Verification items for the finished model (mm, model axes). Face numbers are marked on the shaded views. Give positions to 0.01 mm unless a question says otherwise; leave off trailing zeros. Write each loop counter-clockwise with the first axis right and the second up, starting at its lowest first coordinate (ties: lowest second). Pieces come first, ordered by that corner, then holes.
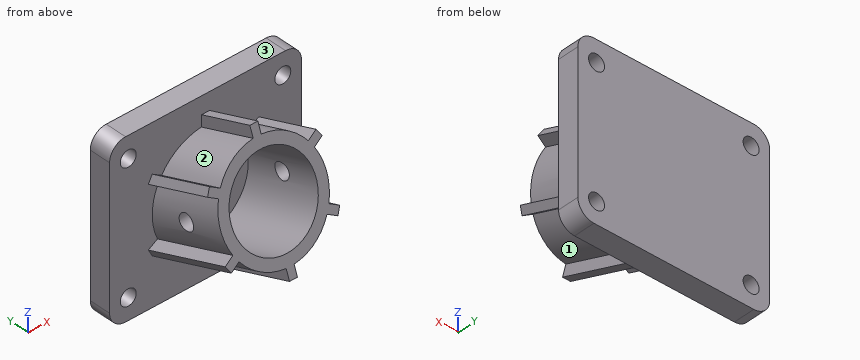
from build123d import *

# Parameters (mm, degrees)
IZIM2_R                     = 1.5
Y_KSEKLIK_EKSTR_ZYON1_DEPTH = 4
Y_KSEKLIK_EKSTR_ZYON2_REACH = 35.135
IZIM4_R                     = 8
KES_EKSTR_ZYON1_REACH       = 45.534
IZIM5_R                     = 1.5


with BuildPart() as part:
    # Çizim2 → Yükseklik-Ekstrüzyon1 (new body)
    with BuildSketch(Plane(origin=(0, 0, 0), x_dir=(1, 0, 0), z_dir=(0, 1, 0))):
        with BuildLine():
            Line((15, -16), (-15, -16))
            ThreePointArc((-15, -16), (-17.121320344, -15.121320344), (-18, -13))
            Line((-18, -13), (-18, 13))
            ThreePointArc((-18, 13), (-17.121320344, 15.121320344), (-15, 16))
            Line((-15, 16), (15, 16))
            ThreePointArc((15, 16), (17.121320344, 15.121320344), (18, 13))
            Line((18, 13), (18, -13))
            ThreePointArc((18, -13), (17.121320344, -15.121320344), (15, -16))
        make_face()
        with Locations(Location((14.5, -12, 0), (0, 0, 270))):
            Circle(IZIM2_R, mode=Mode.SUBTRACT)
        with Locations(Location((-14.5, -12, 0), (0, 0, 270))):
            Circle(IZIM2_R, mode=Mode.SUBTRACT)
        with Locations(Location((14.5, 12, 0), (0, 0, 270))):
            Circle(IZIM2_R, mode=Mode.SUBTRACT)
        with Locations(Location((-14.5, 12, 0), (0, 0, 270))):
            Circle(IZIM2_R, mode=Mode.SUBTRACT)
    extrude(amount=Y_KSEKLIK_EKSTR_ZYON1_DEPTH)

    # Yükseklik-Ekstrüzyon2: up to this plane
    y_kseklik_ekstr_zyon2_end = Plane(origin=(15, 0, -13), z_dir=(0, 1, 0))
    # Çizim4 → Yükseklik-Ekstrüzyon2 (add, up to the surface)
    with BuildSketch(Plane(origin=(0, -14.095389312, 5.13030215), x_dir=(-1, 0, 0), z_dir=(0, -0.9396926207859094, 0.34202014332566627)), mode=Mode.PRIVATE) as y_kseklik_ekstr_zyon2_sk1:
        with BuildLine():
            Line((-0.75, 11.971835338), (-0.75, 9.971835338))
            ThreePointArc((-0.75, 9.971835338), (-5, 8.660254038), (-8.260862725, 5.635436722))
            Line((-8.260862725, 5.635436722), (-9.992913532, 6.635436722))
            Line((-9.992913532, 6.635436722), (-10.742913532, 5.336398616))
            Line((-10.742913532, 5.336398616), (-9.010862725, 4.336398616))
            ThreePointArc((-9.010862725, 4.336398616), (-10, 0), (-9.010862725, -4.336398616))
            Line((-9.010862725, -4.336398616), (-10.742913532, -5.336398616))
            Line((-10.742913532, -5.336398616), (-9.992913532, -6.635436722))
            Line((-9.992913532, -6.635436722), (-8.260862725, -5.635436722))
            ThreePointArc((-8.260862725, -5.635436722), (-5, -8.660254038), (-0.75, -9.971835338))
            Line((-0.75, -9.971835338), (-0.75, -11.971835338))
            Line((-0.75, -11.971835338), (0.75, -11.971835338))
            Line((0.75, -11.971835338), (0.75, -9.971835338))
            ThreePointArc((0.75, -9.971835338), (5, -8.660254038), (8.260862725, -5.635436722))
            Line((8.260862725, -5.635436722), (9.992913532, -6.635436722))
            Line((9.992913532, -6.635436722), (10.742913532, -5.336398616))
            Line((10.742913532, -5.336398616), (9.010862725, -4.336398616))
            ThreePointArc((9.010862725, -4.336398616), (10, 0), (9.010862725, 4.336398616))
            Line((9.010862725, 4.336398616), (10.742913532, 5.336398616))
            Line((10.742913532, 5.336398616), (9.992913532, 6.635436722))
            Line((9.992913532, 6.635436722), (8.260862725, 5.635436722))
            ThreePointArc((8.260862725, 5.635436722), (5, 8.660254038), (0.75, 9.971835338))
            Line((0.75, 9.971835338), (0.75, 11.971835338))
            Line((0.75, 11.971835338), (-0.75, 11.971835338))
        make_face()
        with Locations(Location((0, 0, 0), (0, 0, 90))):
            Circle(IZIM4_R, mode=Mode.SUBTRACT)
    y_kseklik_ekstr_zyon2_tool1 = split(extrude(y_kseklik_ekstr_zyon2_sk1.sketch, amount=-Y_KSEKLIK_EKSTR_ZYON2_REACH, mode=Mode.PRIVATE), bisect_by=y_kseklik_ekstr_zyon2_end, keep=Keep.BOTH, mode=Mode.PRIVATE)
    add(y_kseklik_ekstr_zyon2_tool1.solids().sort_by_distance((-0.428295, -17.847978, -5.179851))[0])

    # Çizim5 → Kes-Ekstrüzyon1 (cut, up to next)
    with BuildSketch(Plane.ZY.offset(18), mode=Mode.PRIVATE) as kes_ekstr_zyon1_sk1:
        with Locations((2.565151075, -7.047694656)):
            Circle(IZIM5_R)
    kes_ekstr_zyon1_tool1 = extrude(kes_ekstr_zyon1_sk1.sketch, amount=-KES_EKSTR_ZYON1_REACH, mode=Mode.PRIVATE) & part.part
    add(kes_ekstr_zyon1_tool1.solids().sort_by_distance((-18, -7.047695, 2.565151))[0], mode=Mode.SUBTRACT)
    add(kes_ekstr_zyon1_tool1.solids().sort_by_distance((-18, -7.047695, 2.565151))[1], mode=Mode.SUBTRACT)


solid = part.part
Item 1: Sectioned sample at B-B on z = -12. Record the cut outline in (x, y).
Answer key:
outline: (-18, 0) - (-16, 0) - (-16, 4) - (-18, 4) - close; (-13, 0) - (-0.75, 0) - (-0.75, -2.03) - (0.75, -2.03) - (0.75, 0) - (13, 0) - (13, 4) - (-13, 4) - close; (16, 0) - (18, 0) - (18, 4) - (16, 4) - close
Item 2: Scan lines: line 1 along X through (y, z) = (2.9, 12); line 2 along Y through (x, z) = (1, 8); line 3 along X through (y, z) = (-14.25, -6). Record each from-to range of solid material in increasing order.
Answer key:
line 1: x = -18 to -16, -13 to 13, 16 to 18
line 2: y = 0 to 4
line 3: x = -0.75 to 0.75
Item 3: Sectioned sample at A-A on x = 14.5. Record the cut outline in (y, z).
Answer key:
outline: (0, -16) - (4, -16) - (4, -13.5) - (0, -13.5) - close; (0, -10.5) - (4, -10.5) - (4, 10.5) - (0, 10.5) - close; (0, 13.5) - (4, 13.5) - (4, 16) - (0, 16) - close
Item 4: Sectioned sample at C-C on x = -6. Record the cut outline in (y, z).
Answer key:
outline: (-16.83, -2.39) - (0, -8.51) - (0, -16) - (4, -16) - (4, 16) - (0, 16) - (0, 8.51) - (-11.36, 12.65) - (-12.29, 10.1) - (0, 5.63) - (0, -5.63) - (-15.91, 0.16) - close
Item 5: Depth check by flat-ended pin: pin 1 (1 mm diameter, centred on y = -14.5, z = 2, fed in from +X); pin 2 (4 mm diameter, centred on x = -1, z = 12.5, fed in from -Y); pin 3 (3 mm diameter, centred on y = -6.5, z = 12, fed in from +X); pin 4 (13 mm diameter, centred on x = 3.5, z = -3.5, fed in from -Y). Enter the tip coordinate at first touch or a pass-through.
Answer key:
pin 1: stops at x = 9.66
pin 2: stops at y = -11.55
pin 3: stops at x = 6.55
pin 4: stops at y = -18.19
Item 6: Release check for a two-part mould opening along Y. For the marked faces 1, 2 and 3 record: released by +Y, released by -Y, zero draft, split by the parting line, or undercut.
Answer key:
face 1: released by -Y
face 2: undercut
face 3: zero draft
Item 7: Sectioned sample at D-D on z = 12. State how many separate pieces and enclosed holes the cut face has, then the cut area to 3 significant figures.
Answer key:
separate pieces: 3
enclosed holes: 0
area: 191 mm2
